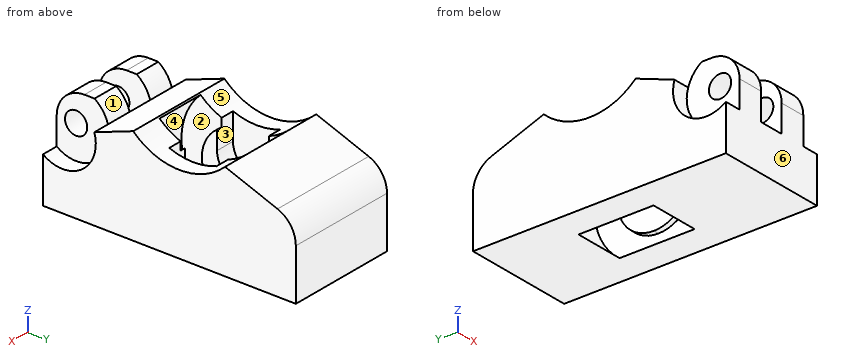
from build123d import *

# Parameters (mm, degrees)
BOSS_EXTRU_1_DEPTH      = 20
ENL_V_MAT_EXTRU_1_REACH = 22
ESQUISSE2_R             = 2
ESQUISSE2_R_2           = 12
ENL_V_START             = -3
ENL_V_MAT_EXTRU_7_DEPTH = 14
CONG_1_R                = 5
ESQUISSE5_R             = 11.25
ENL_V_MAT_EXTRU_2_DEPTH = 4.5
BOSS_EXTRU_2_DEPTH      = 1
ESQUISSE11_R            = 6
ENL_V_MAT_EXTRU_3_DEPTH = 2.25
ENL_V_START_2           = 10
ENL_V_MAT_EXTRU_4_DEPTH = 3
ENL_V_START_3           = -7
ESQUISSE11_3_R          = 6
ENL_V_MAT_EXTRU_5_DEPTH = 3
ENL_V_MAT_EXTRU_6_DEPTH = 20


with BuildPart() as part:
    # Esquisse1 → Boss.-Extru.1 (new body)
    with BuildSketch(Plane(origin=(0, 0, 0), x_dir=(0, 0, -1), z_dir=(1, 0, 0))):
        Polygon((0, 22.75), (0, -22.75), (-18, -22.75), (-18, -8.1), (-18, 8.1), (-12.667836068, 22.75), align=None)
    extrude(amount=BOSS_EXTRU_1_DEPTH)

    # Esquisse2 → Enl_v. mat.-Extru.1 (cut, up to next)
    with BuildSketch(Plane.ZY, mode=Mode.PRIVATE) as enl_v_mat_extru_1_sk1:
        with Locations((13, -19.25)):
            Circle(ESQUISSE2_R)
    enl_v_mat_extru_1_tool1 = extrude(enl_v_mat_extru_1_sk1.sketch, amount=-ENL_V_MAT_EXTRU_1_REACH, mode=Mode.PRIVATE) & part.part
    add(enl_v_mat_extru_1_tool1.solids().sort_by_distance((0, -19.25, 13))[0], mode=Mode.SUBTRACT)
    # Esquisse2 → Enl_v. mat.-Extru.1 (cut, up to next)
    with BuildSketch(Plane.ZY, mode=Mode.PRIVATE) as enl_v_mat_extru_1_sk2:
        with Locations((26, 1.75)):
            Circle(ESQUISSE2_R_2)
    enl_v_mat_extru_1_tool2 = extrude(enl_v_mat_extru_1_sk2.sketch, amount=-ENL_V_MAT_EXTRU_1_REACH, mode=Mode.PRIVATE) & part.part
    add(enl_v_mat_extru_1_tool2.solids().sort_by_distance((0, 1.75, 26))[0], mode=Mode.SUBTRACT)

    # Esquisse14 → Enl_v. mat.-Extru.7 (cut)
    with BuildSketch(Plane.ZY.offset(ENL_V_START)):
        with BuildLine():
            Line((10, 6), (14.777812156, 6))
            ThreePointArc((14.777812156, 6), (14, 1.75), (14.777812156, -2.5))
            Line((14.777812156, -2.5), (10, -2.5))
            ThreePointArc((10, -2.5), (5.75, 1.75), (10, 6))
        make_face()
    extrude(amount=-ENL_V_MAT_EXTRU_7_DEPTH, mode=Mode.SUBTRACT)

    # Cong_1
    cong_1_edges = [part.edges().sort_by_distance(p)[0] for p in [
        (10, -22.75, 18),
        (10, 22.75, 12.667836068),
    ]]
    fillet(cong_1_edges, radius=CONG_1_R)

    # Esquisse5 → Enl_v. mat.-Extru.2 (cut, symmetric)
    with BuildSketch(Plane.ZY.offset(-10)):
        with Locations((9.002244805, 1.517900266)):
            Circle(ESQUISSE5_R)
    extrude(amount=ENL_V_MAT_EXTRU_2_DEPTH, both=True, mode=Mode.SUBTRACT)

    # Esquisse8 → Boss.-Extru.2 (add)
    with BuildSketch(Plane(origin=(5.5, 0, 0), x_dir=(0, 0, -1), z_dir=(1, 0, 0))):
        with BuildLine():
            Line((-12.461710624, 6), (-10, 6))
            ThreePointArc((-10, 6), (-5.75, 1.75), (-10, -2.5))
            Line((-10, -2.5), (-13.309218442, -2.5))
            ThreePointArc((-13.309218442, -2.5), (-6.034488781, -4.92870357), (-1.509850884, 1.263868155))
            ThreePointArc((-1.509850884, 1.263868155), (-5.429840061, 7.229900685), (-12.461710624, 6))
        make_face()
    boss_extru_2 = extrude(amount=BOSS_EXTRU_2_DEPTH)

    # Sym_trie1: Boss.-Extru.2 across plane
    add(boss_extru_2.mirror(Plane.ZY.offset(-10)))

    # Esquisse11 → Enl_v. mat.-Extru.3 (cut, symmetric)
    with BuildSketch(Plane.ZY.offset(-10)):
        with Locations((13, -19.25)):
            Circle(ESQUISSE11_R)
    extrude(amount=ENL_V_MAT_EXTRU_3_DEPTH, both=True, mode=Mode.SUBTRACT)

    # Esquisse11 → Enl_v. mat.-Extru.4 (cut)
    with BuildSketch(Plane.ZY.offset(-10).offset(ENL_V_START_2)):
        with Locations((13, -19.25)):
            Circle(ESQUISSE11_R)
    extrude(amount=-ENL_V_MAT_EXTRU_4_DEPTH, mode=Mode.SUBTRACT)

    # Esquisse11_3 → Enl_v. mat.-Extru.5 (cut)
    with BuildSketch(Plane.ZY.offset(-10).offset(ENL_V_START_3)):
        with Locations((13, -19.25)):
            Circle(ESQUISSE11_3_R)
    extrude(amount=-ENL_V_MAT_EXTRU_5_DEPTH, mode=Mode.SUBTRACT)

    # Esquisse13 → Enl_v. mat.-Extru.6 (cut)
    with BuildSketch(Plane.ZY):
        with BuildLine():
            Line((18, -7.19427191), (17.30217057, -6.517270602))
            Line((17.30217057, -6.517270602), (14.75603403, -13.512723252))
            ThreePointArc((14.75603403, -13.512723252), (16.588298751, -14.441246308), (18, -15.93337521))
            Line((18, -15.93337521), (18, -7.19427191))
        make_face()
    extrude(amount=-ENL_V_MAT_EXTRU_6_DEPTH, mode=Mode.SUBTRACT)


solid = part.part
Could you check a few things on this model? Use its own coordinates, in mm. Face numbers are marked on the shaded views. A direction names the side the tool comes from. Coordinates: 2 decimals unless noted, no trailing zeros. Order: outer loops, then holes, each group sorted by start corner. A loop starts at its lowest first (then second) coordinate and runs counter-clockwise, first axis right, second up.
Q1. Suppose I cut it at A-A on x = 8.25. Please give me the cut outline in (y, z).
Q2. Which directions (+Z, -Z, +X, -X, +Y, -Y) give clear straight access to the entire face, cutting with the end or side of a thin tool? Please do the marked faces 1, 2 and 3.
Q3. Thinking about a two-plate mould opening in Z: for the marked faces 4, 5 and 6, which applies, released by +Z, released by -Z, zero draft, split by the parting line, or undercut?
Q4. Suppose I cut it at D-D on x = 4.75. Please give me the cut outline in (y, z).
Q5. Suppose I cut it at C-C on z = 16. Please give me the cut outline in (x, y), and give its area (3 significant figures).
Q6. Will these pins go through, and if not, where does the flat tip stop? pin 1 (3 mm diameter, centred on x = 4, z = 12.5, fed in from +Y); pin 2 (3 mm diameter, centred on y = -19.5, z = 11, fed in from -X); pin 3 (1.8 mm diameter, centred on x = 15, z = 13, fed in from +Y).
Q7. Suppose I cut it at B-B on y = -8.5. Please give me the cut outline in (x, z), and give its area (3 significant figures).
Q8. Please list where these lines run through material, in increasing order: L1, parallel to X at y = -2, z = 13; L2, parallel to Y at x = 14.7, z = 13; L3, parallel to Y at x = 16.25, z = 13.75.
Answer:
1. outline: (-22.75, 0) - (-5.23, 0) arc R11.25 cw to (-6.3, 17.1) arc R12 cw to (-6.52, 17.3) - (-13.51, 14.76) arc R6 cw to (-22.75, 8.13) - close; (8.26, 0) - (22.75, 0) - (22.75, 9.17) arc R5 ccw to (19.46, 13.87) - (10.02, 17.3) arc R12 cw to (9.55, 16.88) arc R11.25 cw to start
2. face 1: +Z, +X, -X
2. face 2: none
2. face 3: +Z
3. face 4: undercut
3. face 5: released by +Z
3. face 6: zero draft
4. outline: (-22.75, 0) - (22.75, 0) - (22.75, 9.17) arc R5 ccw to (19.46, 13.87) - (10.02, 17.3) arc R12 cw to (6, 14.78) - (6, 10) arc R4.25 cw to (-2.5, 10) - (-2.5, 14.78) arc R12 cw to (-6.52, 17.3) - (-13.51, 14.76) arc R6 ccw to (-15.93, 18) - (-17.75, 18) arc R5 ccw to (-22.75, 13) - close; hole circle Ø4 at (-19.25, 13)
5. outline: (0, -10.09) - (20, -10.09) - (20, -4.88) - (14.5, -4.88) - (14.5, -7.29) - (5.5, -7.29) - (5.5, -4.88) - (0, -4.88) - close; (0, 8.38) - (5.5, 8.38) - (5.5, 10.33) - (14.5, 10.33) - (14.5, 8.38) - (20, 8.38) - (20, 13.59) - (0, 13.59) - close; (3, -21.75) - (7.75, -21.75) - (7.75, -14.05) - (3, -14.05) - close; (12.25, -21.75) - (17, -21.75) - (17, -14.05) - (12.25, -14.05) - close
5. area: 242 mm2
6. pin 1: stops at y = 22.4
6. pin 2: stops at x = 3
6. pin 3: stops at y = 21.8
7. outline: (0, 0) - (20, 0) - (20, 16.58) - (0, 16.58) - close; hole (5.5, 3.88) - (14.5, 3.88) - (14.5, 14.12) - (5.5, 14.12) - close
7. area: 239 mm2
8. L1: x = 0 to 3, 17 to 20
8. L2: y = -22.75 to -21.25, -17.25 to -2.5, 6 to 20.96
8. L3: y = -22.69 to -21.1, -17.4 to -2.5, 6 to 19.75
